from build123d import *

# Parameters (mm, degrees)
F0_R     = 11.05
F1_DEPTH = 7.62


with BuildPart() as f1:
    # F0 (on Top) → F1 (new body)
    with BuildSketch(Plane.XY):
        Polygon((0, 52.410126), (-8.458121, 52.410126), (-19.045388, 35.357095), (-15.727155, 12.67334), (-18.839012, 7.283446), (-40.142837, -1.184758), (-49.617561, -18.880115), (-45.3885, -26.205063), (-41.15944, -33.53001), (-21.097449, -34.172338), (-3.111857, -19.956786), (3.111857, -19.956786), (21.097449, -34.172338), (41.15944, -33.53001), (45.3885, -26.205063), (49.617561, -18.880115), (40.142837, -1.184758), (18.839012, 7.283446), (15.727155, 12.67334), (19.045388, 35.357095), (8.458121, 52.410126), align=None)
        with Locations((-29.759655, -17.181745)):
            Circle(F0_R, mode=Mode.SUBTRACT)
        with Locations((29.759655, -17.181745)):
            Circle(F0_R, mode=Mode.SUBTRACT)
        Circle(F0_R, mode=Mode.SUBTRACT)
        with Locations((0, 34.363489)):
            Circle(F0_R, mode=Mode.SUBTRACT)
    extrude(amount=F1_DEPTH)


solid = f1.part
The model under review builds one solid part; all positions refer to its coordinate system, in mm. A direction names the side the tool comes from. Round coordinates to 2 decimals unless told otherwise and drop trailing zeros. Order: outer loops, then holes, each group sorted by start corner. A loop starts at its lowest first (then second) coordinate and runs counter-clockwise, first axis right, second up. Notation, with made-up numbers: (41.25, 81) -> (78.25, 81) arc R19 cw to (78.25, 111) -> close; hole circle Ø5 at (79.25, 0). An arc over 180 degrees is marked (long way). Write item = value, one per line. Start each with the question number.
Item 1: Clearance check with flat-ended pins moving along their axes: pin 1 Ø1.5 at (x, z) = (0, 4.5) entering from -Y; pin 2 Ø17.5 at (x, y) = (0, 34.36) entering from -Z; pin 3 Ø1 at (y, z) = (-12, 3) entering from +X. State where each tip first meets the part, or that it passes through.
Item 2: Consider section D-D on y = 0. Write out the cut boundary in (x, z).
Item 3: Mouldability with a two-part tool opening along X and no side actions: class faces 1 (the face through (11.979, -26.965, 3.757)), 2 (the face through (10, 10, 0)), 3 (the face through (-29.34, 3.11, 3.76)) as released by +X, released by -X, zero draft, split by the parting line, or undercut.
Item 4: Consider section C-C on y = -9. Write out the cut boundary in (x, z).
Item 5: Consider section B-B on z = 3.5. Write out the cut boundary in (x, y), plus the area to 3 significant figures.
Item 6: For line 1 along Y through (x, z) = (0, 2.5); line 2 along X through (y, z) = (-8.5, 3.5); line 3 along X through (y, z) = (-20, 5.5), list the stretches that pass through material, from the lowest coordinate up.
Item 7: Consider section A-A on x = 0. Write out the cut boundary in (y, z), plus the area to 3 significant figures.
Item 8: For faces 4 (the face through (18.72, -16.7, 3.76)), 5 (the face through (-17.26, 10.02, 3.76)), 6 (the face through (17.305, 9.941, 3.757)), list the 3-axis set-ups (+Z, -Z, +X, -X, +Y, -Y) from which the entire face can be reached by the end or side of a thin tool; tool diameter is ignored.
Conclusion:
q1.pin_1 = -19.96
q1.pin_2 = through
q1.pin_3 = 46.2
q2.outline = (-37.16, 0) -> (-11.05, 0) -> (-11.05, 7.62) -> (-37.16, 7.62) -> close; (11.05, 0) -> (37.16, 0) -> (37.16, 7.62) -> (11.05, 7.62) -> close
q3.face_1 = undercut
q3.face_2 = zero draft
q3.face_3 = released by -X
q4.outline = (-44.33, 0) -> (-37.19, 0) -> (-37.19, 7.62) -> (-44.33, 7.62) -> close; (-22.33, 0) -> (-6.41, 0) -> (-6.41, 7.62) -> (-22.33, 7.62) -> close; (6.41, 0) -> (22.33, 0) -> (22.33, 7.62) -> (6.41, 7.62) -> close; (37.19, 0) -> (44.33, 0) -> (44.33, 7.62) -> (37.19, 7.62) -> close
q5.outline = (-49.62, -18.88) -> (-41.16, -33.53) -> (-21.1, -34.17) -> (-3.11, -19.96) -> (3.11, -19.96) -> (21.1, -34.17) -> (41.16, -33.53) -> (49.62, -18.88) -> (40.14, -1.18) -> (18.84, 7.28) -> (15.73, 12.67) -> (19.05, 35.36) -> (8.46, 52.41) -> (-8.46, 52.41) -> (-19.05, 35.36) -> (-15.73, 12.67) -> (-18.84, 7.28) -> (-40.14, -1.18) -> close; hole circle Ø22.1 at (-29.76, -17.18); hole circle Ø22.1 at (0, 0); hole circle Ø22.1 at (0, 34.36); hole circle Ø22.1 at (29.76, -17.18)
q5.area = 3,020 mm2
q6.line_1 = -19.96 to -11.05, 11.05 to 23.31, 45.41 to 52.41
q6.line_2 = -44.06 to -36.6, -22.92 to -7.06, 7.06 to 22.92, 36.6 to 44.06
q6.line_3 = -48.97 to -40.44, -19.08 to -3.17, 3.17 to 19.08, 40.44 to 48.97
q7.outline = (-19.96, 0) -> (-11.05, 0) -> (-11.05, 7.62) -> (-19.96, 7.62) -> close; (11.05, 0) -> (23.31, 0) -> (23.31, 7.62) -> (11.05, 7.62) -> close; (45.41, 0) -> (52.41, 0) -> (52.41, 7.62) -> (45.41, 7.62) -> close
q7.area = 215 mm2
q8.face_4 = +Z, -Z
q8.face_5 = +Z, -Z, -X
q8.face_6 = +Z, -Z, +X
